Input: dimensioned drawing with shaded views. Units: mm. Origin: part minimum x, y, z. A direction names the side the tool comes from. Coordinates: 2 decimals unless noted, no trailing zeros. Loops run counter-clockwise (first coordinate to the right, second up) from the corner with the lowest first, then second, coordinate; pieces in that order, holes last. Notation, with made-up numbers: (85, -36.5) -> (128, -36.5) arc R27 cw to (128, -2.5) -> close; hole circle Ø7 at (37.5, 7). An arc over 180 degrees is marked (long way). Answer as CSV lines item,"result".
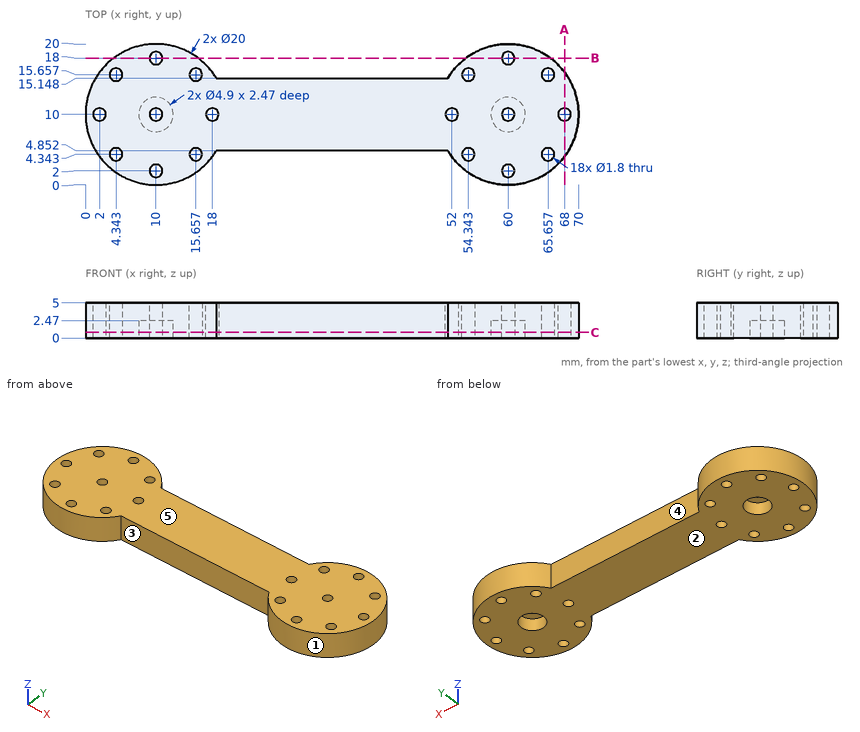
(1) Access query for the marked faces 3, 4 and 5. Directions: +Z, -Z, +X, -X, +Y, -Y. A direction counts if a zero-diameter tool reaches every point of the face in a straight line with its end or side. Return the directions, or none.
Computed values:
face 3,"+Z, -Z, -Y"
face 4,"+Z, -Z, +Y"
face 5,"+Z, +X, -X, +Y, -Y"
(2) Pin query (flat end, axial travel): pin 1 Ø1.1 at (x, y) = (10, 10) entering from -Z; pin 2 Ø1.5 at (x, y) = (9, 9.5) entering from -Z. Return the tip coordinate at first contact, or that it passes through.
Computed values:
pin 1,"through"
pin 2,"z = 2.47"
(3) Draft query along X for the marked faces 1 and 2. Return one class per face: released by +X, released by -X, zero draft, split by the parting line, or undercut.
Computed values:
face 1,"undercut"
face 2,"zero draft"
(4) Cut plane C-C (z = 0.8). State how many separate pieces and enclosed holes the cut face has, then the cut area to 3 significant figures.
Computed values:
separate pieces,"1"
enclosed holes,"18"
area,"868 mm^2"
(5) Material intervals for L1, parallel to Y at x = 10, z = 3.5; L2, parallel to Y at x = 60, z = 1.45; L3, parallel to X at y = 11.75, z = 1.55 (1 decimal), sorted ascending. Write a range as [from, to].
Computed values:
L1,"[0, 1.1], [2.9, 9.1], [10.9, 17.1], [18.9, 20]"
L2,"[0, 1.1], [2.9, 7.55], [12.45, 17.1], [18.9, 20]"
L3,"[0.2, 8.3], [11.7, 58.3], [61.7, 69.8]"
(6) Cut plane A-A (x = 68). Return the cut outline in (y, z), then the cut area to 3 significant figures.
Computed values:
outline,"(4, 0) -> (9.1, 0) -> (9.1, 5) -> (4, 5) -> close; (10.9, 0) -> (16, 0) -> (16, 5) -> (10.9, 5) -> close"
area,"51.0 mm^2"
(7) Cut plane B-B (y = 18). Return the cut outline in (x, z).
Computed values:
outline,"(4, 0) -> (9.1, 0) -> (9.1, 5) -> (4, 5) -> close; (10.9, 0) -> (16, 0) -> (16, 5) -> (10.9, 5) -> close; (54, 0) -> (59.1, 0) -> (59.1, 5) -> (54, 5) -> close; (60.9, 0) -> (66, 0) -> (66, 5) -> (60.9, 5) -> close"
